Input: part model. Units: mm. Frame: model coordinates. A direction names the side the tool comes from. Round coordinates to 2 decimals unless told otherwise and drop trailing zeros. Use one line per item in the form item = value. Start each with the question number.
Q1. First-contact query: P1, Ø3, axis at y = -1, z = 2, coming from the +X side. Flat tip, straight axial feed; report the tip coordinate or a pass-through.
Q2. Access query for faces 1 (the flat face through (0, 18, 2)), 2 (the flat face through (6.35, 2.2, 0.3)), 3 (the cylindrical face through (5.55, -69.76, 117.4)). Directions: +Z, -Z, +X, -X, +Y, -Y. A direction counts if a zero-diameter tool reaches every point of the face in a straight line with its end or side. Return the directions, or none.
Q3. Ray query, line 1 along Y through (x, z) = (11.25, -114.3); line 2 along Y through (x, z) = (12.25, -2); line 3 along X through (y, z) = (-72.25, -114.3). Return the intervals inside material, ascending.
Q4. Mould query, pull axis Z, two halves, no side actions, for faces 4 (the flat face through (6, -1, -127)), 5 (the flat face through (6.35, 0, 114)), 6 (the flat face through (6, -1, 127)). Classes: pulls with the +Z half, pulls with the -Z half, needs draft (parallel to the pull), parting line crosses it, or undercut.
```python
from build123d import *

# Parameters (mm, degrees)
SKETCH1_W                       = 254
SKETCH1_H                       = 152.4
BOSS_EXTRUDE1_DEPTH             = 12.7
SKETCH3_R                       = 6.35
CUT_EXTRUDE2_DEPTH              = 6.35
F_1_4_0_25_DIAMETER_HOLE1_D     = 6.35
F_1_4_0_25_DIAMETER_HOLE1_DEPTH = 12.7
F_1_4_0_25_DIAMETER_HOLE1_TIP   = 1.907732465
SKETCH7_W                       = 38.1
SKETCH7_H                       = 9.652
CUT_EXTRUDE3_DEPTH              = 6.35


with BuildPart() as part:
    # Sketch1 → Boss-Extrude1 (new body)
    with BuildSketch(Plane(origin=(0, 0, 0), x_dir=(0, 0, -1), z_dir=(1, 0, 0))):
        Rectangle(SKETCH1_W, SKETCH1_H)
    extrude(amount=BOSS_EXTRUDE1_DEPTH)

    # Sketch3 → Cut-Extrude2 (cut)
    with BuildSketch(Plane(origin=(12.7, 0, 0), x_dir=(0, 0, -1), z_dir=(1, 0, 0))):
        with Locations((114.3, 0)):
            Circle(SKETCH3_R)
        with Locations((-114.3, 0)):
            Circle(SKETCH3_R)
    extrude(amount=-CUT_EXTRUDE2_DEPTH, mode=Mode.SUBTRACT)

    # 1/4 (0.25) Diameter Hole1
    with Locations(Plane(origin=(0, -76.2, 0), x_dir=(-1, 0, 0), z_dir=(0, -1, 0))):
        with Locations((-6.236337014, -114.3), (-6.236337014, 0), (-6.236337014, 114.3)):
            Hole(F_1_4_0_25_DIAMETER_HOLE1_D / 2, depth=F_1_4_0_25_DIAMETER_HOLE1_DEPTH)
            with Locations((0, 0, -(F_1_4_0_25_DIAMETER_HOLE1_DEPTH + F_1_4_0_25_DIAMETER_HOLE1_TIP / 2))):  # 118° drill point
                Cone(0, F_1_4_0_25_DIAMETER_HOLE1_D / 2, F_1_4_0_25_DIAMETER_HOLE1_TIP, mode=Mode.SUBTRACT)

    # Sketch7 → Cut-Extrude3 (cut)
    with BuildSketch(Plane(origin=(12.7, 0, 0), x_dir=(0, 0, -1), z_dir=(1, 0, 0))):
        Rectangle(SKETCH7_W, SKETCH7_H)
    extrude(amount=-CUT_EXTRUDE3_DEPTH, mode=Mode.SUBTRACT)

    # Sketch10 → #10-32 Tapped Hole1 (revolve, cut)
    with BuildSketch(Plane(origin=(6.35, 0, 0), x_dir=(0, 0, -1), z_dir=(0, 1, 0))):
        Polygon((0, 0), (0, 6.35), (2.6543, 6.35), (2.0193, 5.715), (2.0193, 0), align=None)
    revolve(axis=Axis((12.7, 0, 0), (-1, 0, 0)), mode=Mode.SUBTRACT)


solid = part.part
```
Results found:
q1.P1 = 6.35
q2.face_1 = +Z, -Z, -X, +Y, -Y
q2.face_2 = +X
q2.face_3 = -Y
q3.line_1 = -76.2 to -6.35, 6.35 to 76.2
q3.line_2 = -76.2 to -4.83, 4.83 to 76.2
q3.line_3 = 0 to 3.06, 9.41 to 12.7
q4.face_4 = pulls with the -Z half
q4.face_5 = undercut
q4.face_6 = pulls with the +Z half
